Geometry check sheet. Reference: the model listing, model coordinates, mm. A direction names the side the tool comes from. Give positions to 0.01 mm unless a question says otherwise; leave off trailing zeros. Order: outer loops, then holes, each group sorted by start corner. A loop starts at its lowest first (then second) coordinate and runs counter-clockwise, first axis right, second up. Notation, with made-up numbers: M 83.5,44 L 118.5,44 A28 cw 118.5,69 Z; hole C 47,82 d3. An arc over 180 degrees is marked long. Use CSV: the item, a comma, the result in double quotes. Start each with the question number.
from build123d import *

# Parameters (mm, degrees)
SKETCH1_W           = 1119
SKETCH1_H           = 70
BOSS_EXTRUDE1_DEPTH = 46.8
SKETCH2_W           = 86.6
SKETCH2_H           = 70
BOSS_EXTRUDE2_DEPTH = 185.4
SKETCH4_R           = 2.75
CUT_EXTRUDE1_DEPTH  = 10


with BuildPart() as part:
    # Sketch1 → Boss-Extrude1 (new body)
    with BuildSketch(Plane(origin=(0, 0, 0), x_dir=(1, 0, 0), z_dir=(0, 1, 0))):
        Rectangle(SKETCH1_W, SKETCH1_H)
    extrude(amount=BOSS_EXTRUDE1_DEPTH)

    # Sketch2 → Boss-Extrude2 (add)
    with BuildSketch(Plane.XZ):
        with Locations((602.8, 0)):
            Rectangle(SKETCH2_W, SKETCH2_H)
    extrude(amount=-BOSS_EXTRUDE2_DEPTH)

    # Sketch4 → Cut-Extrude1 (cut)
    with BuildSketch(Plane(origin=(0, 46.8, 0), x_dir=(1, 0, 0), z_dir=(0, 1, 0))):
        with Locations((92.478641365, 22)):
            Circle(SKETCH4_R)
        with Locations((92.478641365, -22)):
            Circle(SKETCH4_R)
    extrude(amount=-CUT_EXTRUDE1_DEPTH, mode=Mode.SUBTRACT)


solid = part.part
(1) Thickness scan on line 1 (X direction, y = 43.5, z = -22); line 2 (Y direction, x = -15, z = 3); line 3 (X direction, y = 128, z = 27.5). Record the ranges inside material, lowest first.
(2) Go/stop test with flat-tipped pins: P1, Ø12, axis at x = -99, z = -5.5, coming from the +Y side; P2, Ø1.5, axis at y = 151.5, z = 21.5, coming from the -X side; P3, Ø1.6, axis at x = 92.5, z = 22, coming from the +Y side. Record where each tip stops, or that it passes through.
(3) Access from +Z, -Z, +X, -X, +Y, -Y to the whole of each face (thin tool, end or side, straight path). Record for faces 1 (the face through (646.1, 91, 0)), 2 (the face through (-8, 46.8, 0)).
(4) Sectioned sample at C-C on x = 373.5. Record the cut outline in (y, z).
(5) Sectioned sample at B-B on y = 80.5. Record the cut outline in (x, z), then the cut area to 3 significant figures.
(6) Sectioned sample at A-A on z = -3.5. Record the cut outline in (x, y), then the cut area to 3 significant figures.
Responses:
1,line 1,"-559.5 to 89.73, 95.23 to 646.1"
1,line 2,"0 to 46.8"
1,line 3,"559.5 to 646.1"
2,P1,"y = 46.8"
2,P2,"x = 559.5"
2,P3,"y = 36.8"
3,face 1,"+Z, -Z, +X, +Y, -Y"
3,face 2,"+Z, -Z, -X, +Y"
4,outline,"M 0,-35 L 46.8,-35 L 46.8,35 L 0,35 Z"
5,outline,"M 559.5,-35 L 646.1,-35 L 646.1,35 L 559.5,35 Z"
5,area,"6,060 mm2"
6,outline,"M -559.5,0 L 646.1,0 L 646.1,185.4 L 559.5,185.4 L 559.5,46.8 L -559.5,46.8 Z"
6,area,"68,400 mm2"
